Autodesk Inventor part; units mm, degrees
ref_plane "YZ Plane" through (0, 0, 0) normal (1, 0, 0) x (0, 1, 0)
ref_plane "XZ Plane" through (0, 0, 0) normal (0, 1, 0) x (-1, 0, 0)
ref_plane "XY Plane" through (0, 0, 0) normal (0, 0, 1) x (1, 0, 0)
sketch "Sketch1" plane through (0, 0, 0) normal (0, 1, 0) x (-1, 0, 0)
  line L0 (-55, 55) -> (55, 55)
  line L1 (55, 55) -> (55, -55)
  line L2 (55, -55) -> (-55, -55)
  line L3 (-55, -55) -> (-55, 55)
  line L4 (-55, 55) -> (55, -55) construction
  line L5 (55, 55) -> (-55, -55) construction
  line L6 (-12.5, 37.5) -> (12.5, 37.5) construction
  line L7 (12.5, 37.5) -> (12.5, -37.5) construction
  line L8 (12.5, -37.5) -> (-12.5, -37.5) construction
  line L9 (-12.5, -37.5) -> (-12.5, 37.5) construction
  line L10 (-12.5, 37.5) -> (12.5, -37.5) construction
  line L11 (12.5, 37.5) -> (-12.5, -37.5) construction
  line L12 (-37.5, 37.5) -> (37.5, 37.5) construction
  line L13 (37.5, 37.5) -> (37.5, -37.5) construction
  line L14 (37.5, -37.5) -> (-37.5, -37.5) construction
  line L15 (-37.5, -37.5) -> (-37.5, 37.5)
  line L16 (-37.5, 37.5) -> (37.5, -37.5) construction
  line L17 (37.5, 37.5) -> (-37.5, -37.5) construction
  circle A0 centre (37.5, -37.5) radius 2 construction
  circle A1 centre (37.5, 37.5) radius 2 construction
  circle A2 centre (-37.5, 37.5) radius 2 construction
  circle A3 centre (-37.5, -37.5) radius 2 construction
  point P0 (0, 0)
  dimension "d0" = 110
  dimension "d1" = 110
  dimension "d2" = 25
  dimension "d3" = 75
  dimension "d4" = 75
  dimension "d5" = 4
  dimension "d6" = 4
  dimension "d7" = 4
  dimension "d8" = 4
extrude "Extrusion1" add sketch "Sketch1" along normal blind 3
sketch "Sketch3" plane through (0, 3, 0) normal (0, 1, 0) x (1, 0, 0)
  line L0 (35, -35) -> (-35, -35)
  line L1 (-35, -35) -> (-35, 35)
  line L2 (-35, 35) -> (35, 35)
  line L3 (35, 35) -> (35, -35)
  line L4 (35, -35) -> (-35, 35) construction
  line L5 (-35, -35) -> (35, 35) construction
  point P0 (0, 0)
  dimension "d18" = 70
  dimension "d19" = 70
extrude "Extrusion3" [suppressed]
fillet "Fillet1" [suppressed]
sketch "Sketch4" plane through (0, 3, 0) normal (0, 1, 0) x (1, 0, 0)
  line L0 (28, -16) -> (42, -16)
  line L1 (42, -16) -> (42, 16)
  line L2 (42, 16) -> (28, 16)
  line L3 (28, 16) -> (28, -16)
  line L4 (28, -16) -> (42, 16) construction
  line L5 (42, -16) -> (28, 16) construction
  line L6 (35, 33) -> (35, -33)
  point P0 (0, 0)
  point P1 (35, 0)
  dimension "d23" = 14
  dimension "d24" = 32
extrude "Extrusion4" [suppressed]
sketch "Sketch5" plane through (0, 3, 0) normal (0, 1, 0) x (1, 0, 0)
  line L0 (-30, -11.5) -> (30, -11.5)
  line L1 (30, -11.5) -> (30, 11.5)
  line L2 (30, 11.5) -> (-30, 11.5)
  line L3 (-30, 11.5) -> (-30, -11.5)
  line L4 (-30, -11.5) -> (30, 11.5) construction
  line L5 (30, -11.5) -> (-30, 11.5) construction
  point P0 (0, 0)
  dimension "d31" = 23
  dimension "d32" = 60
extrude "Extrusion5" cut sketch "Sketch5" against normal blind 10
sketch "Sketch6" plane through (0, 3, 0) normal (0, 1, 0) x (1, 0, 0)
  line L0 (-38.5, 13.25) -> (38.5, 13.25)
  line L1 (38.5, 13.25) -> (38.5, -13.25)
  line L2 (38.5, -13.25) -> (-38.5, -13.25)
  line L3 (-38.5, -13.25) -> (-38.5, 13.25)
  line L4 (-38.5, 13.25) -> (38.5, -13.25) construction
  line L5 (38.5, 13.25) -> (-38.5, -13.25) construction
  point P0 (0, 0)
  dimension "d35" = 26.5
  dimension "d36" = 77
extrude "Extrusion6" cut sketch "Sketch6" against normal blind 1
sketch "Sketch7" plane through (0, 3, 0) normal (0, 1, 0) x (1, 0, 0)
  line L0 (-42.5, -20) -> (42.5, -20) construction
  line L1 (42.5, -20) -> (42.5, 20) construction
  line L2 (42.5, 20) -> (-42.5, 20) construction
  line L3 (-42.5, 20) -> (-42.5, -20) construction
  line L4 (-42.5, -20) -> (42.5, 20) construction
  line L5 (42.5, -20) -> (-42.5, 20) construction
  circle A0 centre (-42.5, 20) radius 1
  circle A1 centre (42.5, 20) radius 1
  circle A2 centre (42.5, -20) radius 1
  circle A3 centre (-42.5, -20) radius 1
  point P0 (0, 0)
  dimension "d39" = 40
  dimension "d40" = 85
  dimension "d41" = 2
  dimension "d42" = 2
  dimension "d43" = 2
  dimension "d44" = 2
extrude "Extrusion7" cut sketch "Sketch7" against normal through all
sketch "Sketch8" plane through (0, 3, 0) normal (0, 1, 0) x (1, 0, 0)
  line L0 (55, -55) -> (55, 55)
  line L1 (-55, 55) -> (55, 55)
  line L2 (55, 55) -> (55, -55)
  line L3 (55, -55) -> (-55, -55)
  line L4 (-55, -55) -> (-55, 55)
  line L5 (-55, 55) -> (55, -55) construction
  line L6 (55, 55) -> (-55, -55) construction
  line L7 (-60, 60) -> (60, 60)
  line L8 (60, 60) -> (60, -60)
  line L9 (60, -60) -> (-60, -60)
  line L10 (-60, -60) -> (-60, 60)
  line L11 (-60, 60) -> (60, -60) construction
  line L12 (60, 60) -> (-60, -60) construction
  point P0 (0, 0)
  dimension "d47" = 5
extrude "Extrusion8" add sketch "Sketch8" against normal blind 13.45
sketch "Sketch9" plane through (0, -10.45, 0) normal (0, -1, 0) x (1, 0, 0)
  line L0 (-55, 55) -> (55, 55)
  circle A0 centre (-55, 55) radius 3.5
  line L1 (55, 55) -> (55, -55)
  circle A1 centre (55, 55) radius 3.5
  line L2 (55, -55) -> (-55, -55)
  circle A2 centre (55, -55) radius 3.5
  circle A3 centre (-55, -55) radius 3.5
  point P0 (0, 0)
  dimension "d50" = 7
  dimension "d51" = 7
  dimension "d52" = 7
  dimension "d53" = 7
extrude "Extrusion9" add sketch "Sketch9" against normal blind 13.45
fillet "Fillet3" radius 5 4 edges at (60, -3.725, -60) (60, -3.725, 60) (-60, -3.725, -60) (-60, -3.725, 60)
sketch "Sketch10" plane through (0, -10.45, 0) normal (0, -1, 0) x (1, 0, 0)
  arc A0 (-55, 51.5) -> (-51.5, 55) centre (-55, 55) ccw
  circle A1 centre (-55, 55) radius 1.45
  arc A2 (51.5, 55) -> (55, 51.5) centre (55, 55) ccw
  circle A3 centre (55, 55) radius 1.45
  arc A4 (55, -51.5) -> (51.5, -55) centre (55, -55) ccw
  circle A5 centre (55, -55) radius 1.45
  arc A6 (-51.5, -55) -> (-55, -51.5) centre (-55, -55) ccw
  circle A7 centre (-55, -55) radius 1.45
  point P0 (0, 0)
  dimension "d57" = 2.9
  dimension "d58" = 2.9
  dimension "d59" = 2.9
  dimension "d60" = 2.9
extrude "Extrusion10" cut sketch "Sketch10" against normal blind 13.45
sketch "Sketch11" plane through (0, 3, 0) normal (0, 1, 0) x (1, 0, 0)
  circle A0 centre (-55, 55) radius 1.45
  circle A1 centre (-55, 55) radius 3
  circle A2 centre (55, 55) radius 1.45
  circle A3 centre (55, 55) radius 3
  circle A4 centre (55, -55) radius 1.45
  circle A5 centre (55, -55) radius 3
  circle A6 centre (-55, -55) radius 1.45
  circle A7 centre (-55, -55) radius 3
  point P0 (0, 0)
  dimension "d63" = 6
  dimension "d64" = 6
  dimension "d65" = 6
  dimension "d66" = 6
extrude "Extrusion11" cut sketch "Sketch11" against normal blind 1.8 contours A0 | A1 | A2 | A3 | A5 | A7
properties part number "3D printed box top"
Part model, mm, in its own coordinate system. A direction names the side the tool comes from. Round coordinates to 2 decimals unless told otherwise and drop trailing zeros. Write each loop counter-clockwise with the first axis right and the second up, starting at its lowest first coordinate (ties: lowest second). Pieces come first, ordered by that corner, then holes. Notation, with made-up numbers: (69, 56.5) -> (84, 56.5) arc R15 ccw to (84, 69.5) -> close; hole circle Ø10 at (49, 30). An arc over 180 degrees is marked (long way). Return JSON: item names as keys, results as strings. Group by question number.
Q1. Saw through at C-C on y = -4.75. Write the cut outline in (x, z).
Q2. Saw through at A-A on x = -2. Write the cut outline in (y, z).
Q3. Saw through at D-D on x = -33. Write the cut outline in (y, z).
Q4. Pin check, flat tips, straight feed: pin 1 (2.5 mm diameter, centred on x = 55, z = 55, fed in from +Y); pin 2 (5 mm diameter, centred on x = 0, z = 21, fed in from -Y); pin 3 (1.8 mm diameter, centred on x = -54.5, z = -53.5, fed in from +Y). Stop position of each tip, or through.
Q5. Which spindle directions (+Z, -Z, +X, -X, +Y, -Y) get a long thin tool onto all of the face, cutting with end or side? Do faces 1 (the cylindrical face through (-59, -4, -58)), 2 (the cylindrical face through (52.55, -5.3, -52.5)). Say none if no direction does.
Q6. Mould opens along Z. For faces 3 (the cylindrical face through (-52.5, -5.3, -52.55)), 4 (the cylindrical face through (-52.55, -5.3, 52.5)), 5 (the flat face through (-1, -4, -60)), 6 (the flat face through (0, -10.45, -58)) say: pulls with the +Z half, pulls with the -Z half, needs draft (parallel to the pull), parting line crosses it, or undercut.
Q7. Saw through at B-B on z = 25.5. Write the cut outline in (x, y), plus the area to 4 significant figures.
Q8. Probe L1, parallel to X at y = 2, z = -55; L2, parallel to X at y = 1.3, z = -20; L3, parallel to Z at x = -42.5, y = 1.4. List the from-to ranges inside material, lowest first. Write a range as [from, to].
Answer:
{
 "1": {"outline": "(-60, -55) arc R5 ccw to (-55, -60) -> (55, -60) arc R5 ccw to (60, -55) -> (60, 55) arc R5 ccw to (55, 60) -> (-55, 60) arc R5 ccw to (-60, 55) -> close; hole circle Ø2.9 at (-55, -55); hole circle Ø2.9 at (-55, 55); hole (-55, -51.5) arc R3.5 cw to (-51.5, -55) -> (51.5, -55) arc R3.5 cw to (55, -51.5) -> (55, 51.5) arc R3.5 cw to (51.5, 55) -> (-51.5, 55) arc R3.5 cw to (-55, 51.5) -> close; hole circle Ø2.9 at (55, -55); hole circle Ø2.9 at (55, 55)"},
 "2": {"outline": "(-10.45, -60) -> (3, -60) -> (3, -13.25) -> (2, -13.25) -> (2, -11.5) -> (0, -11.5) -> (0, -55) -> (-10.45, -55) -> close; (-10.45, 55) -> (0, 55) -> (0, 11.5) -> (2, 11.5) -> (2, 13.25) -> (3, 13.25) -> (3, 60) -> (-10.45, 60) -> close"},
 "3": {"outline": "(-10.45, -60) -> (3, -60) -> (3, -13.25) -> (2, -13.25) -> (2, 13.25) -> (3, 13.25) -> (3, 60) -> (-10.45, 60) -> (-10.45, 55) -> (0, 55) -> (0, -55) -> (-10.45, -55) -> close"},
 "4": {"pin 1": "through", "pin 2": "y = 0", "pin 3": "y = 1.2"},
 "5": {"face 1": "-Z, -X, +Y, -Y", "face 2": "-Y"},
 "6": {"face 3": "undercut", "face 4": "undercut", "face 5": "pulls with the -Z half", "face 6": "needs draft"},
 "7": {"outline": "(-60, -10.45) -> (-55, -10.45) -> (-55, 0) -> (55, 0) -> (55, -10.45) -> (60, -10.45) -> (60, 3) -> (-60, 3) -> close", "area": "464.5 mm2"},
 "8": {"L1": "[-60, -58], [-52, 52], [58, 60]", "L2": "[-60, -43.5], [-41.5, 41.5], [43.5, 60]", "L3": "[-60, -21], [-19, 19], [21, 60]"}
}
